from build123d import *

# Parameters (mm, degrees)
SCHIZZO1_R                  = 6
PIASTRABASE_DEPTH           = 20
SCHIZZO2_R                  = 100
CORPOCILINDRICO_DEPTH       = 120
SCHIZZO3_R                  = 107.5
SCHIZZO4_R                  = 107.5
CORPOCILINDRICOFINALE_DEPTH = 12.3
PANNELLOCOMANDI_DEPTH       = 125


with BuildPart() as part:
    # Schizzo1 → PiastraBase (new body)
    with BuildSketch(Plane.XY):
        with BuildLine():
            Line((-80, -100), (80, -100))
            ThreePointArc((80, -100), (94.142135624, -94.142135624), (100, -80))
            Line((100, -80), (100, 80))
            ThreePointArc((100, 80), (94.142135624, 94.142135624), (80, 100))
            Line((80, 100), (-80, 100))
            ThreePointArc((-80, 100), (-94.142135624, 94.142135624), (-100, 80))
            Line((-100, 80), (-100, -80))
            ThreePointArc((-100, -80), (-94.142135624, -94.142135624), (-80, -100))
        make_face()
        with Locations((-80, 80)):
            Circle(SCHIZZO1_R, mode=Mode.SUBTRACT)
        with Locations(Location((-80, -80, 0), (0, 0, 180))):
            Circle(SCHIZZO1_R, mode=Mode.SUBTRACT)
        with Locations((80, -80)):
            Circle(SCHIZZO1_R, mode=Mode.SUBTRACT)
        with Locations(Location((80, 80, 0), (0, 0, 180))):
            Circle(SCHIZZO1_R, mode=Mode.SUBTRACT)
    extrude(amount=PIASTRABASE_DEPTH)

    # Schizzo2 → CorpoCilindrico (add)
    with BuildSketch(Plane.XY.offset(20)):
        Circle(SCHIZZO2_R)
    extrude(amount=CORPOCILINDRICO_DEPTH)

    # Schizzo3 → section 1 of loftcentrale
    with BuildSketch(Plane.XY.offset(190.7), mode=Mode.PRIVATE) as loftcentrale_s1:
        Circle(SCHIZZO3_R)
    # loft up to a face of the part (loftcentrale)
    loft([Face(Wire([part.edges().sort_by_distance((-68.454710593, 72.896862742, 140))[0]])), loftcentrale_s1.sketch])

    # Schizzo4 → CorpoCilindricoFinale (add)
    with BuildSketch(Plane.XY.offset(190.7)):
        Circle(SCHIZZO4_R)
    extrude(amount=CORPOCILINDRICOFINALE_DEPTH)

    # Schizzo5 → PannelloComandi (add)
    with BuildSketch(Plane.XY):
        with BuildLine():
            Line((-95.684335707, 56), (-139.684335707, 56))
            Line((-139.684335707, 56), (-139.684335707, -56))
            Line((-139.684335707, -56), (-95.684335707, -56))
            Line((-95.684335707, -56), (-74.684335707, -66.5))
            ThreePointArc((-74.684335707, -66.5), (-93.45703176, -35.577847246), (-100, 0))
            ThreePointArc((-100, 0), (-93.45703176, 35.577847246), (-74.684335707, 66.5))
            Line((-74.684335707, 66.5), (-95.684335707, 56))
        make_face()
    extrude(amount=PANNELLOCOMANDI_DEPTH)


solid = part.part
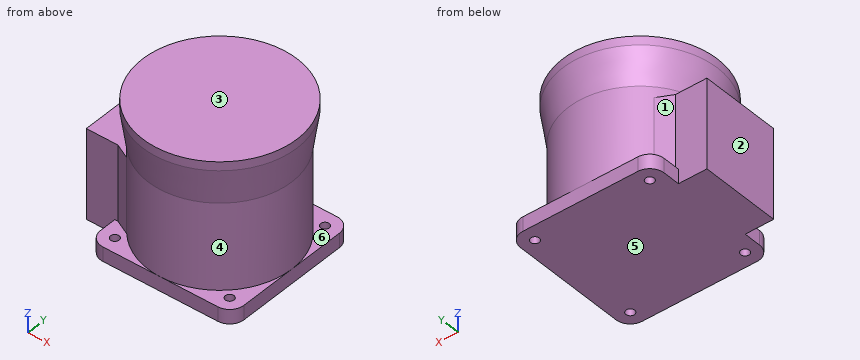
Could you check a few things on this model? Use its own coordinates, in mm. Face numbers are marked on the shaded views. A direction names the side the tool comes from. Coordinates: 2 decimals unless noted, no trailing zeros. Order: outer loops, then holes, each group sorted by start corner. A loop starts at its lowest first (then second) coordinate and runs counter-clockwise, first axis right, second up.
Q1. Will these pins go through, and if not, where does the flat tip stop? pin 1 (9.5 mm diameter, centred on x = -80, y = 80, fed in from +Z); pin 2 (8 mm diameter, centred on x = -51, z = 151, fed in from -Y); pin 3 (2 mm diameter, centred on x = -10.5, z = 127, fed in from -Y); pin 4 (10 mm diameter, centred on y = -24, z = 7, fed in from +X).
Q2. Suppose I cut it at A-A on z = 77.5. Please give me the cut outline in (x, y).
Q3. Thinking about a two-plate mould opening in Z: for the marked faces 1, 2 and 3, which applies, released by +Z, released by -Z, zero draft, split by the parting line, or undercut?
Q4. Suppose I cut it at B-B on x = -118. Please give me the cut outline in (y, z), and give its area (3 significant figures).
Q5. Which directions (+Z, -Z, +X, -X, +Y, -Y) give clear straight access to the entire face, cutting with the end or side of a thin tool? Please do the marked faces 4, 5 and 6.
Q6. Please list where these lines run through material, in increasing order: L1, parallel to Y at x = -80, z = 9.5; L2, parallel to Y at x = -113, z = 110; L3, parallel to Z at x = -59.5, y = 98.
Answer:
1. pin 1: passes through
1. pin 2: stops at y = -90.21
1. pin 3: stops at y = -99.55
1. pin 4: stops at x = 100
2. outline: (-139.68, -56) - (-95.68, -56) - (-74.68, -66.5) arc R100 ccw (long way) to (-74.68, 66.5) - (-95.68, 56) - (-139.68, 56) - close
3. face 1: undercut
3. face 2: zero draft
3. face 3: released by +Z
4. outline: (-56, 0) - (56, 0) - (56, 125) - (-56, 125) - close
4. area: 14,000 mm2
5. face 4: none
5. face 5: -Z, +X, -X, +Y, -Y
5. face 6: +X, +Y
6. L1: y = -100 to -86, -74 to 74, 86 to 100
6. L2: y = -56 to 56
6. L3: z = 0 to 20
